Verification items for this drawing (mm, ordinates from the low corner). Give positions to 0.01 mm unless a question says otherwise; leave off trailing zeros. Loops run counter-clockwise (first coordinate to the right, second up) from the corner with the lowest first, then second, coordinate; pieces in that order, holes last. Notation, with made-up numbers: M 36,70.25 L 81,70.25 A33 cw 81,104.25 Z; hole C 56,14.5 d5. An arc over 180 degrees is marked long. Put each result on its own line as item: value. Start each with the question number.
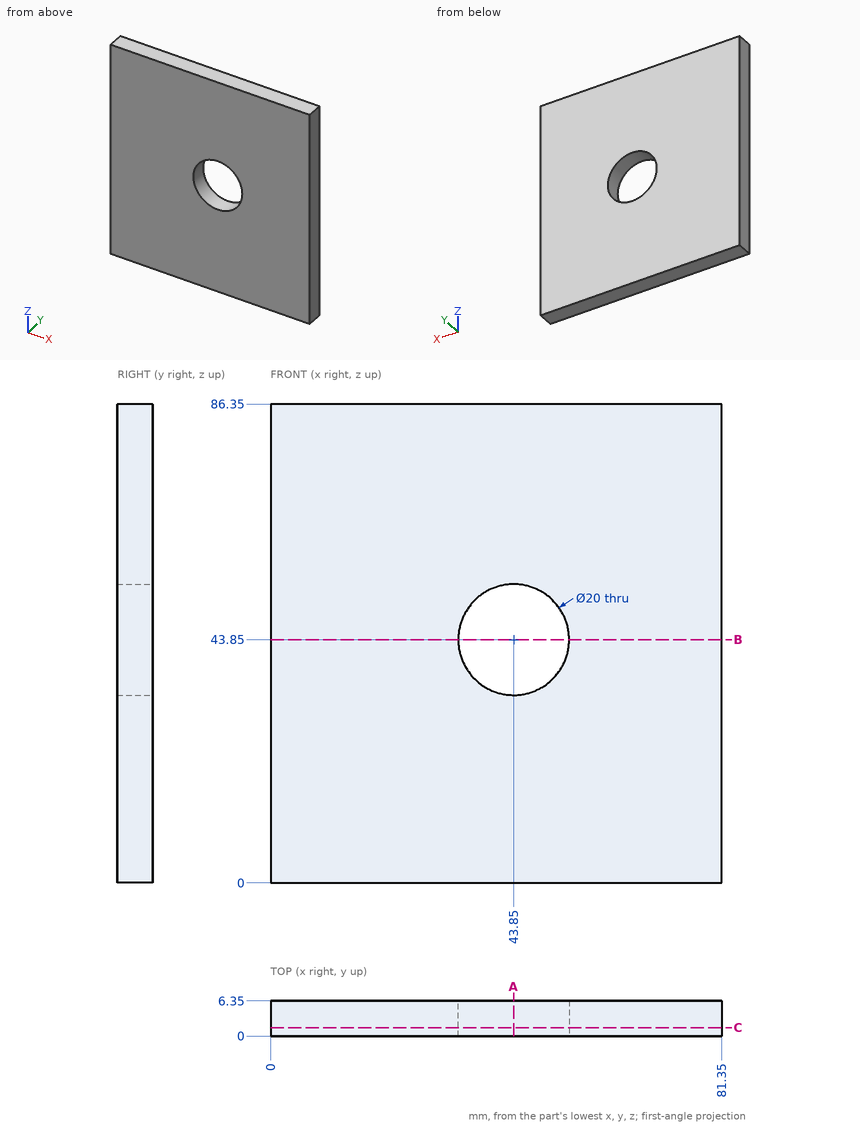
Q1. Cross-section at A-A, the plane x = 43.85. Record the boundary of the cut face in (y, z).
Q2. Cross-section at B-B, the plane z = 43.85. Record the boundary of the cut face in (x, y), then the cut area to 3 significant figures.
Q3. Cross-section at C-C, the plane y = 1.5. Record the boundary of the cut face in (x, z).
Q4. Scan lines: L1, parallel to Z at x = 43.85, y = 4; L2, parallel to X at y = 3, z = 39; L3, parallel to Z at x = 50.5, y = 4. Record each from-to range of solid material in increasing order.
Ans:
1. outline: M 0,0 L 6.35,0 L 6.35,33.85 L 0,33.85 Z; M 0,53.85 L 6.35,53.85 L 6.35,86.35 L 0,86.35 Z
2. outline: M 0,0 L 33.85,0 L 33.85,6.35 L 0,6.35 Z; M 53.85,0 L 81.35,0 L 81.35,6.35 L 53.85,6.35 Z
2. area: 390 mm^2
3. outline: M 0,0 L 81.35,0 L 81.35,86.35 L 0,86.35 Z; hole C 43.85,43.85 d20
4. L1: z = 0 to 33.85, 53.85 to 86.35
4. L2: x = 0 to 35.1, 52.6 to 81.35
4. L3: z = 0 to 36.38, 51.32 to 86.35
